Model file for the job. Use its own axes, mm. A direction names the side the tool comes from. Coordinates: 2 decimals unless noted, no trailing zeros. Write each loop counter-clockwise with the first axis right and the second up, starting at its lowest first coordinate (ties: lowest second). Pieces come first, ordered by that corner, then holes. Notation, with made-up numbers: (-2.5, 11.5) -> (28.5, 11.5) arc R20 ccw to (28.5, 45.5) -> close; hole circle Ø9 at (-24.5, 52.5). An arc over 180 degrees is marked (long way). Answer as a JSON object with one key per item and string values. Group by question number.
from build123d import *

# Parameters (mm, degrees)
F0_R         = 9.525
F1_DEPTH     = 25.4
F2_W         = 19.05
F2_H         = 19.05
F3_DEPTH     = 3.175
F4_T1_DEPTH  = 25.4
F4_T3_DEPTH  = 12.7
F4_T5_DEPTH  = 12.7
F4_S9_W      = 3.175
F4_S9_H      = 3.175
F4_T10_DEPTH = 3.175
F4_S15_W     = 3.175
F4_S15_H     = 3.175
F4_T16_DEPTH = 3.175
F4_S21_W     = 3.175
F4_S21_H     = 3.175
F4_T22_DEPTH = 3.175
F4_S27_W     = 3.175
F4_S27_H     = 3.175
F4_T28_DEPTH = 3.175
F4_T31_DEPTH = 30.3662191739
F5_R         = 1.5875


# Not quite as in the source:
# - a fillet or chamfer that OpenCascade refuses, or shapes differently, is made with other operations: its cross-section is extruded or revolved along the edge and cut away or added


with BuildPart() as f1:
    # F0 (on Right) → F1 (new body)
    with BuildSketch(Plane.YZ):
        with BuildLine():
            Line((16.51, 15.875), (-16.51, 15.875))
            ThreePointArc((-16.51, 15.875), (-29.7854143214, -18.9198974706), (0, -41.275))
            ThreePointArc((0, -41.275), (14.2378547718, -18.3786670428), (-12.5944842771, -15.7359123145))
            ThreePointArc((-12.5944842771, -15.7359123145), (-21.4720341133, -4.1780442704), (-16.51, 9.525))
            Line((-16.51, 9.525), (16.51, 9.525))
            ThreePointArc((16.51, 9.525), (19.685, 12.7), (16.51, 15.875))
        make_face()
        with BuildLine():
            ThreePointArc((-14.343097751, -32.2037615996), (-25.3220142156, -19.7737801421), (-25.6780404598, -3.1932406127))
            ThreePointArc((-25.6780404598, -3.1932406127), (-22.8730710881, -13.3775496244), (-15.115016679, -20.5469704521))
            ThreePointArc((-15.115016679, -20.5469704521), (-15.8403068596, -26.4489535701), (-14.343097751, -32.2037615996))
        make_face(mode=Mode.SUBTRACT)
        with Locations((0, -25.4)):
            Circle(F0_R, mode=Mode.SUBTRACT)
    extrude(amount=F1_DEPTH)

    # F2 (on face) → F3 (cut)
    with BuildSketch(Plane.XY.offset(15.875)):
        with Locations((12.7, 0)):
            Rectangle(F2_W, F2_H)
    extrude(amount=-F3_DEPTH, mode=Mode.SUBTRACT)

    # F4: fillet of radius 3.175 on 11 edges, made by hand

    # F4_s2 → F4_t1 (join)
    with BuildSketch(Plane.YZ):
        with BuildLine():
            ThreePointArc((-15.229163377, 9.525), (-16.4906498384, 9.2636363719), (-17.5444470536, 8.5225760049))
            ThreePointArc((-17.5444470536, 8.5225760049), (-17.0391316289, 9.0360765162), (-16.51, 9.525))
            Line((-16.51, 9.525), (-15.229163377, 9.525))
        make_face()
        with BuildLine():
            ThreePointArc((-15.0737959989, -14.3545542957), (-13.0077413525, -14.9014210416), (-11.0631237972, -14.0147939479))
            ThreePointArc((-11.0631237972, -14.0147939479), (-11.8600660646, -14.8475378256), (-12.5944842771, -15.7359123145))
            ThreePointArc((-12.5944842771, -15.7359123145), (-13.8665248674, -15.1033585978), (-15.0737959989, -14.3545542957))
        make_face()
    extrude(amount=F4_T1_DEPTH)

    # F4_s4 → F4_t3 (join)
    with BuildSketch(Plane.YZ.offset(6.35)):
        with BuildLine():
            ThreePointArc((9.525, 15.875), (8.5950640303, 13.6299359697), (6.35, 12.7))
            Line((6.35, 12.7), (9.525, 12.7))
            Line((9.525, 12.7), (9.525, 15.875))
        make_face()
        with BuildLine():
            ThreePointArc((-9.525, 15.875), (-8.5950640303, 13.6299359697), (-6.35, 12.7))
            Line((-6.35, 12.7), (-9.525, 12.7))
            Line((-9.525, 12.7), (-9.525, 15.875))
        make_face()
    extrude(amount=F4_T3_DEPTH)

    # F4_s6 → F4_t5 (join)
    with BuildSketch(Plane.XZ.offset(-6.35)):
        with BuildLine():
            ThreePointArc((3.175, 15.875), (4.1049359697, 13.6299359697), (6.35, 12.7))
            Line((6.35, 12.7), (3.175, 12.7))
            Line((3.175, 12.7), (3.175, 15.875))
        make_face()
        with BuildLine():
            ThreePointArc((22.225, 15.875), (21.2950640303, 13.6299359697), (19.05, 12.7))
            Line((19.05, 12.7), (22.225, 12.7))
            Line((22.225, 12.7), (22.225, 15.875))
        make_face()
    extrude(amount=F4_T5_DEPTH)


with BuildPart() as f4_tool8:
    # F4_s9 → F4_t10 (new body)
    with BuildSketch(Plane.XY.offset(15.875)):
        with Locations((20.6375, 7.9375)):
            Rectangle(F4_S9_W, F4_S9_H)
    extrude(amount=-F4_T10_DEPTH)

    # F4_s11 → F4_t12 (revolve, cut)
    with BuildSketch(Plane(origin=(19.05, 6.35, 15.875), x_dir=(-0.7071067812, -0.7071067812, 0), z_dir=(0.7071067812, -0.7071067812, 0))):
        with BuildLine():
            ThreePointArc((0, -3.175), (3.175, 0), (0, 3.175))
            Line((0, 3.175), (0, -3.175))
        make_face()
    revolve(axis=Axis((19.05, 6.35, 15.875), (0, 0, -1)), mode=Mode.SUBTRACT)


with BuildPart() as f1_1:
    add(f1.part)

    # F4_t7: union F4_tool8
    add(f4_tool8.part)


with BuildPart() as f4_tool14:
    # F4_s15 → F4_t16 (new body)
    with BuildSketch(Plane.XY.offset(15.875)):
        with Locations((4.7625, 7.9375)):
            Rectangle(F4_S15_W, F4_S15_H)
    extrude(amount=-F4_T16_DEPTH)

    # F4_s17 → F4_t18 (revolve, cut)
    with BuildSketch(Plane(origin=(6.35, 6.35, 15.875), x_dir=(0.7071067812, -0.7071067812, 0), z_dir=(0.7071067812, 0.7071067812, 0))):
        with BuildLine():
            ThreePointArc((0, -3.175), (3.175, 0), (0, 3.175))
            Line((0, 3.175), (0, -3.175))
        make_face()
    revolve(axis=Axis((6.35, 6.35, 15.875), (0, 0, -1)), mode=Mode.SUBTRACT)


with BuildPart() as f1_2:
    add(f1_1.part)

    # F4_t13: union F4_tool14
    add(f4_tool14.part)


with BuildPart() as f4_tool20:
    # F4_s21 → F4_t22 (new body)
    with BuildSketch(Plane.XY.offset(15.875)):
        with Locations((4.7625, -7.9375)):
            Rectangle(F4_S21_W, F4_S21_H)
    extrude(amount=-F4_T22_DEPTH)

    # F4_s23 → F4_t24 (revolve, cut)
    with BuildSketch(Plane(origin=(6.35, -6.35, 15.875), x_dir=(0.7071067812, 0.7071067812, 0), z_dir=(-0.7071067812, 0.7071067812, 0))):
        with BuildLine():
            ThreePointArc((0, -3.175), (3.175, 0), (0, 3.175))
            Line((0, 3.175), (0, -3.175))
        make_face()
    revolve(axis=Axis((6.35, -6.35, 15.875), (0, 0, -1)), mode=Mode.SUBTRACT)


with BuildPart() as f1_3:
    add(f1_2.part)

    # F4_t19: union F4_tool20
    add(f4_tool20.part)


with BuildPart() as f4_tool26:
    # F4_s27 → F4_t28 (new body)
    with BuildSketch(Plane.XY.offset(15.875)):
        with Locations((20.6375, -7.9375)):
            Rectangle(F4_S27_W, F4_S27_H)
    extrude(amount=-F4_T28_DEPTH)

    # F4_s29 → F4_t30 (revolve, cut)
    with BuildSketch(Plane(origin=(19.05, -6.35, 15.875), x_dir=(-0.7071067812, 0.7071067812, 0), z_dir=(-0.7071067812, -0.7071067812, 0))):
        with BuildLine():
            ThreePointArc((0, -3.175), (3.175, 0), (0, 3.175))
            Line((0, 3.175), (0, -3.175))
        make_face()
    revolve(axis=Axis((19.05, -6.35, 15.875), (0, 0, -1)), mode=Mode.SUBTRACT)


with BuildPart() as f1_4:
    add(f1_3.part)

    # F4_t25: union F4_tool26
    add(f4_tool26.part)

    # F4_s32 → F4_t31 (cut)
    with BuildSketch(Plane.YZ.offset(-2.483109587)):
        with BuildLine():
            ThreePointArc((-15.5690922553, 15.875), (-16.4962795763, 15.7366015003), (-17.3426345609, 15.3334716042))
            ThreePointArc((-17.3426345609, 15.3334716042), (-16.9284902387, 15.6075768645), (-16.51, 15.875))
            Line((-16.51, 15.875), (-15.5690922553, 15.875))
        make_face()
    extrude(amount=F4_T31_DEPTH, mode=Mode.SUBTRACT)

    # F5
    f5_edges = [f1_4.edges().sort_by_distance(p)[0] for p in [
        (12.7, -9.525, 15.875),
        (3.175, 0, 15.875),
        (12.7, 9.525, 15.875),
        (22.225, 0, 15.875),
        (12.7, -15.115017, -20.54697),
        (12.7, -14.343098, -32.203762),
        (12.7, -25.67804, -3.193241),
        (21.295064, 8.595064, 15.875),
        (21.295064, -8.595064, 15.875),
        (4.104936, 8.595064, 15.875),
        (4.104936, -8.595064, 15.875),
    ]]
    fillet(f5_edges, radius=F5_R)


solid = f1_4.part
(1) Cut at C-C on z = 2. List the corners of the cut face in (x, y).
(2) 3-axis set-ups, long thin cutter, end or side, ignore diameter. For faces 5 (the face through (12.5, -13, -14.9)), 6 (the face through (13, 0, 9.525)), 7 (the face through (12.61, 8.21, 13.3)), 8 (the face through (13, 11, 15.875)): which of +Z, -Z, +X, -X, +Y, -Y reach the whole face in a straight line?
(3) Cut at B-B on x = 10.25. Give the number of separate pieces and of enclosed holes in the cut face, plus the area to 3 significant figures.
(4) Wall check: probe 1 along Z at (x, y) = (16, 0) (3 decimals); probe 2 along Z at (x, y) = (21.5, -17.5); probe 3 along Y at (x, z) = (5.5, -25.5). Give the ranges that are in metal, low to high.
(5) Pull direction Z, two halves, no side cores. Call faces 1 (the face through (0, -5, -12)), 2 (the face through (12.61, -8.21, 13.3)), 3 (the face through (12.52, -29.8, -18.87)), 4 (the face through (12.52, -24.36, -21.92)): released by +Z, released by -Z, zero draft, split by the parting line, or undercut.
(6) Cut at A-A on z = -25.4. List the corners of the cut face in (x, y) (3 decimals).
(7) Pin check, flat tips, straight feed: pin 1 (3 mm diameter, centred on x = 11, y = -5.5, fed in from +Z); pin 2 (6 mm diameter, centred on x = 4, z = -8.5, fed in from +Y); pin 3 (2 mm diameter, centred on x = 8.5, y = -25.5, fed in from +Z). Stop position of each tip, or through.
(8) Cut at D-D on z = -4.5. List the corners of the cut face in (x, y), plus the area to 3 significant figures.
Results found:
{
 "1": {"outline": "(0, -28.44) -> (25.4, -28.44) -> (25.4, -21.15) -> (0, -21.15) -> close"},
 "2": {"face 5": "+X, -X", "face 6": "+X, -X, +Y", "face 7": "+Z", "face 8": "+Z, +X, -X, +Y, -Y"},
 "3": {"separate pieces": "1", "enclosed holes": "2", "area": "1,080 mm²"},
 "4": {"probe 1": "z = -41.275 to -34.925, -15.875 to -9.525, 9.525 to 12.7", "probe 2": "z = -35.89 to -29.93, -19.12 to -12.28, 8.57 to 15.23", "probe 3": "y = -27.03 to -22.13, -15.87 to -9.52, 9.52 to 15.87"},
 "5": {"face 1": "zero draft", "face 2": "released by +Z", "face 3": "split by the parting line", "face 4": "undercut"},
 "6": {"outline": "(0, -27.084) -> (25.4, -27.084) -> (25.4, -22.203) -> (0, -22.203) -> close; (0, -15.875) -> (25.4, -15.875) -> (25.4, -9.525) -> (0, -9.525) -> close; (0, 9.525) -> (25.4, 9.525) -> (25.4, 15.875) -> (0, 15.875) -> close"},
 "7": {"pin 1": "stops at z = 12.77", "pin 2": "stops at y = 7.67", "pin 3": "stops at z = 8.64"},
 "8": {"outline": "(0, -30.45) -> (25.4, -30.45) -> (25.4, -21.42) -> (0, -21.42) -> close", "area": "229 mm²"}
}
